The listing builds one solid part. Answer for the finished solid, in the listing's coordinates (mm). Coordinates: 2 decimals unless noted, no trailing zeros. Answer as a JSON object with one key per item and string values. Group by question number.
from build123d import *

# Parameters (mm, degrees)
SKETCH1_R           = 486.25
BOSS_EXTRUDE1_DEPTH = 65
SKETCH3_R           = 441.25
CUT_EXTRUDE1_DEPTH  = 35
SKETCH6_R           = 100
BOSS_EXTRUDE3_DEPTH = 55
BOSS_EXTRUDE4_DEPTH = 25
CIRPATTERN1_COUNT   = 9


with BuildPart() as part:
    # Sketch1 → Boss-Extrude1 (new body)
    with BuildSketch(Plane(origin=(0, 0, 0), x_dir=(1, 0, 0), z_dir=(0, 1, 0))):
        Circle(SKETCH1_R)
    extrude(amount=BOSS_EXTRUDE1_DEPTH)

    # Sketch3 → Cut-Extrude1 (cut)
    with BuildSketch(Plane(origin=(0, 65, 0), x_dir=(1, 0, 0), z_dir=(0, 1, 0))):
        Circle(SKETCH3_R)
    extrude(amount=-CUT_EXTRUDE1_DEPTH, mode=Mode.SUBTRACT)

    # Sketch5 → Cut-Revolve1 (revolve, cut)
    with BuildSketch(Plane(origin=(0, 0, 0), x_dir=(0, 0, -1), z_dir=(1, 0, 0))):
        Polygon((486.25, 45), (478.929491924, 17.679491924), (461.25, 0), (486.25, 0), align=None)
    revolve(axis=Axis((0, 89.25, 0), (0, -1, 0)), mode=Mode.SUBTRACT)

    # Sketch6 → Boss-Extrude3 (add)
    with BuildSketch(Plane(origin=(0, 30, 0), x_dir=(1, 0, 0), z_dir=(0, 1, 0))):
        Circle(SKETCH6_R)
    extrude(amount=BOSS_EXTRUDE3_DEPTH)

    # Sketch7 → Boss-Extrude4 (add)
    with BuildSketch(Plane(origin=(0, 30, 0), x_dir=(1, 0, 0), z_dir=(0, 1, 0))):
        with BuildLine():
            Line((0, 441.25), (0, 100))
            ThreePointArc((0, 100), (13.767464211, 99.047750753), (27.272727273, 96.209138584))
            ThreePointArc((27.272727273, 96.209138584), (22.022759648, 99.799825551), (20, 105.830052443))
            Line((20, 105.830052443), (20, 430.205256244))
            ThreePointArc((20, 430.205256244), (23.179315347, 437.518139456), (30.695652174, 440.181030302))
            ThreePointArc((30.695652174, 440.181030302), (15.357129929, 440.982676599), (0, 441.25))
        make_face()
        with BuildLine():
            Line((-20, 372.762072239), (-20, 105.830052443))
            ThreePointArc((-20, 105.830052443), (-22.022759648, 99.799825551), (-27.272727273, 96.209138584))
            ThreePointArc((-27.272727273, 96.209138584), (-13.767464211, 99.047750753), (0, 100))
            Line((0, 100), (0, 441.25))
            ThreePointArc((0, 441.25), (-46.554925044, 438.787193813), (-92.590163934, 431.426267214))
            ThreePointArc((-92.590163934, 431.426267214), (-42.286672356, 419.427958259), (-20, 372.762072239))
        make_face()
    boss_extrude4 = extrude(amount=BOSS_EXTRUDE4_DEPTH)

    # CirPattern1: Boss-Extrude4 ×9 about axis
    cirpattern1_axis = Axis((0, 0, 0), (0, 1, 0))
    for i in range(1, CIRPATTERN1_COUNT):
        add(boss_extrude4.rotate(cirpattern1_axis, i * 360 / CIRPATTERN1_COUNT))


solid = part.part
Item 1: Consider L1, parallel to Z at x = 0, y = 54; L2, parallel to X at y = 49, z = 212.5; L3, parallel to Y at x = 142.5, z = -316. Determine where each line is inside the solid, lowest interval first. Write a range as from..to.
Item 2: For a pull along X with two mould halves and no side action, classify faces 1 (the face through (-42.872, 42.325, -419.895)), 2 (the face through (463.796, 54.86, -146.056)), 3 (the face through (-6, 0, -6)) as +X half, -X half, draft (parallel to the pull), parting line (faces both ways), or undercut.
Item 3: Flat-ended cylindrical pins translate along their axes: pin 1 Ø1.5 at (y, z) = (68.5, -55) entering from -X; pin 2 Ø5 at (x, y) = (-16, 20.5) entering from -Z; pin 3 Ø6 at (x, y) = (-90.5, 68.5) entering from +Z. Find the tip coordinate at first contact, or state that the pin passes through.
Answer:
{
 "1": {"L1": "-486.25..100, 441.25..486.25", "L2": "-437.36..-324.5, -98.63..-56.06, 56.06..98.63, 328.06..437.36", "L3": "0..30"},
 "2": {"face 1": "undercut", "face 2": "parting line", "face 3": "draft"},
 "3": {"pin 1": "x = -84.01", "pin 2": "z = -480.09", "pin 3": "z = 48.41"}
}
